CAD build for the part. Positions are in the model's coordinates, mm. A direction names the side the tool comes from. Give positions to 0.01 mm unless a question says otherwise; leave off trailing zeros. Write each loop counter-clockwise with the first axis right and the second up, starting at its lowest first coordinate (ties: lowest second). Pieces come first, ordered by that corner, then holes. Notation, with made-up numbers: (63.25, 29) -> (69.25, 29) arc R9 cw to (69.25, 40) -> close; hole circle Ø6 at (-16, 18). An arc over 180 degrees is marked (long way). Answer as a JSON object with one key per item and string values.
Autodesk Inventor part; units mm, degrees
ref_plane "YZ Plane" through (0, 0, 0) normal (1, 0, 0) x (0, 1, 0)
ref_plane "XZ Plane" through (0, 0, 0) normal (0, 1, 0) x (-1, 0, 0)
ref_plane "XY Plane" through (0, 0, 0) normal (0, 0, 1) x (1, 0, 0)
sketch "Náčrt1" plane through (0, 0, 0) normal (0, 0, 1) x (1, 0, 0)
  line L0 (43, 17) -> (26, 0)
  line L1 (43, 17) -> (43, 43)
  line L2 (29, 130) -> (43, 43)
  line L3 (26, 0) -> (13, 0)
  line L4 (29, 130) -> (13, 130)
  line L5 (13, 134.5754) -> (13, -3.2687)
  line L6 (-17, 17) -> (0, 0)
  line L7 (-17, 17) -> (-17, 43)
  line L8 (-3, 130) -> (-17, 43)
  line L9 (0, 0) -> (13, 0)
  line L10 (-3, 130) -> (13, 130)
  dimension "d3" = 26
  dimension "d6" = 13
  dimension "d7" = 16
extrude "Vysunutí1" add sketch "Náčrt1" along normal blind 40
sketch "Náčrt2" plane through (43, 17, 0) normal (1, 0, 0) x (0, 0, -1)
  line L0 (0, 113) -> (-40, 113)
  line L1 (-28, 113) -> (-28, 53)
  line L2 (-28, 53) -> (-12, 53)
  line L3 (-12, 53) -> (-12, 113)
  line L4 (-28, 113) -> (-12, 113)
  point P0 (0, -17)
  dimension "d10" = 60
  dimension "d11" = 16
extrude "Vysunutí2" cut sketch "Náčrt2" against normal through all
sketch "Náčrt3" plane through (0, 0, 40) normal (0, 0, 1) x (1, 0, 0)
  circle A0 centre (13, 30) radius 20
  circle A1 centre (13, 110) radius 10
  point P0 (0, 0)
  dimension "d14" = 40
  dimension "d15" = 20
extrude "Vysunutí3" cut sketch "Náčrt3" against normal through all contours A0
sketch "Náčrt4" plane through (0, 0, 40) normal (0, 0, 1) x (1, 0, 0)
  circle A0 centre (13, 110) radius 10
  point P0 (0, 0)
  dimension "d18" = 20
extrude "Vysunutí4" cut sketch "Náčrt4" against normal blind 20
properties part number "11"
1) Slice it at D-D (x = 13). List the corners of the cut face in (y, z), then the cut area to 3 significant figures.
Model answer:
{"outline": "(0, 0) -> (10, 0) -> (10, 40) -> (0, 40) -> close; (50, 0) -> (130, 0) -> (130, 12) -> (70, 12) -> (70, 28) -> (100, 28) -> (100, 40) -> (50, 40) -> close; (120, 28) -> (130, 28) -> (130, 40) -> (120, 40) -> close", "area": "2,400 mm2"}
2) Slice it at B-B (y = 30). List the corners of the cut face in (x, z), then the cut area to 3 significant figures.
Model answer:
{"outline": "(-17, 0) -> (-7, 0) -> (-7, 40) -> (-17, 40) -> close; (33, 0) -> (43, 0) -> (43, 40) -> (33, 40) -> close", "area": "800 mm2"}
3) Wall check: probe 1 along Y at (x, z) = (13, 33.5); probe 2 along Z at (x, y) = (20.5, 75); probe 3 along Y at (x, z) = (13, 27.5). Give the ranges that are in metal, low to high.
Model answer:
{"probe 1": "y = 0 to 10, 50 to 100, 120 to 130", "probe 2": "z = 0 to 12, 28 to 40", "probe 3": "y = 0 to 10, 50 to 70"}
4) Mould opens along Y. For faces 1 (the flat face through (13, 0, 20)), 2 (the cylindrical face through (-1.74, 43.52, 20.28)), 3 (the flat face through (13, 94, 28)), 4 (the flat face through (-9.9, 87.11, 10.83)) say: released by +Y, released by -Y, zero draft, split by the parting line, or undercut.
Model answer:
{"face 1": "released by -Y", "face 2": "undercut", "face 3": "zero draft", "face 4": "released by +Y"}
5) 3-axis set-ups, long thin cutter, end or side, ignore diameter. For faces 5 (the flat face through (13, 70, 20)), 6 (the flat face through (-9, 9, 20)), 7 (the cylindrical face through (11.698, 119.915, 34.084)): which of +Z, -Z, +X, -X, +Y, -Y reach the whole face in a straight line?
Model answer:
{"face 5": "+X, -X, +Y", "face 6": "+Z, -Z, -X, -Y", "face 7": "+Z"}
6) Pin check, flat tips, straight feed: pin 1 (1.5 mm diameter, centred on y = 99.5, z = 27.5, fed in from +X); pin 2 (6 mm diameter, centred on y = 85, z = 25.5, fed in from +X); pin 3 (23 mm diameter, centred on x = 13, y = 110, fed in from -Z); pin 4 (5 mm diameter, centred on x = 10.5, z = 19, fed in from +Y). Stop position of each tip, or through.
Model answer:
{"pin 1": "stops at x = 34", "pin 2": "stops at x = 36.51", "pin 3": "stops at z = 0", "pin 4": "stops at y = 70"}
7) Slice it at C-C (z = 36). List the corners of the cut face in (x, y), then the cut area to 3 significant figures.
Model answer:
{"outline": "(-17, 17) -> (0, 0) -> (26, 0) -> (43, 17) -> (43, 43) -> (29, 130) -> (-3, 130) -> (-17, 43) -> close; hole circle Ø40 at (13, 30); hole circle Ø20 at (13, 110)", "area": "4,720 mm2"}
8) Slice it at A-A (z = 24.5). List the corners of the cut face in (x, y), then the cut area to 3 significant figures.
Model answer:
{"outline": "(-17, 17) -> (0, 0) -> (26, 0) -> (43, 17) -> (43, 43) -> (38.66, 70) -> (-12.66, 70) -> (-17, 43) -> close; hole circle Ø40 at (13, 30)", "area": "2,540 mm2"}
